For this review, take the finished solid that the model builds, in its own axes (mm). A direction names the side the tool comes from. Round coordinates to 2 decimals unless told otherwise and drop trailing zeros. Order: outer loops, then holes, each group sorted by start corner. A loop starts at its lowest first (then second) coordinate and runs counter-clockwise, first axis right, second up. Notation, with made-up numbers: (80.5, -10) -> (132.5, -10) arc R24 cw to (132.5, 3) -> close; hole circle Ø6 at (-32.75, 81.5). An arc over 180 degrees is marked (long way). Use a Markdown table: item, result. Add a question column.
1) Draft analysis for pull direction Y (two halves, no side actions). For faces 5 (the face through (29.65, 0, 16)), 6 (the face through (0, -18.5, 16)), 7 (the face through (-32, 0, 16)), state which applies: pulls with the +Y half, pulls with the -Y half, needs draft (parallel to the pull), parting line crosses it, or undercut.
2) Consider section B-B (z = 37). State the section outline as (x, y) points, plus the area to 3 significant figures.
3) Machinability: for faces 1 (the face through (30.841, 0.199, 15.496)), 2 (the face through (0, 0, 27)), 3 (the face through (-14, 17, 39)), 4 (the face through (31, 2, 2)), which of the approach directions +Z, -Z, +X, -X, +Y, -Y give a long, thin tool a straight path to every point of the face, cutting with its end or side? Answer none if there is none.
4) Wall thickness on line 1 along X through (y, z) = (12.5, 30.25); line 2 along X through (y, z) = (-12, 30); line 3 along Y through (x, z) = (-3, 19): over which ranges is each line inside the solid? List them lowest first. Write a range as [from, to].
5) Clearance check with flat-ended pins moving along their axes: P1, Ø1.5, axis at x = -11.5, y = -12, coming from the -Z side; P2, Ø2.5, axis at x = 30.5, y = 0, coming from the +Z side; P3, Ø3, axis at x = 14, y = 16, coming from the +Z side. State where each tip first meets the part, or that it passes through.
6) Consider section D-D (y = -8). State the section outline as (x, z) points.
7) Consider section C-C (z = 10). State the section outline as (x, y) points.
8) Consider section A-A (x = 17). State the section outline as (y, z) points.
```python
from build123d import *

# Parameters (mm, degrees)
SKETCH_1_W                 = 64
SKETCH_1_H                 = 37
EXTRUDE_1_DEPTH            = 42
SHELL_1_T                  = -2.35
SHELL_1_THICKNESS_2_FACE_W = 59.3
SHELL_1_THICKNESS_2_FACE_H = 32.3
SHELL_1_THICKNESS_2_DEPTH  = 12.65
F_3_0MM_START              = 27
F_3_0MM_1_OUTLINE_R        = 1.3
F_3_0MM_1_DEPTH            = 15
SKETCH_4_R                 = 18
CUT_EXTRUDE_1_DEPTH        = 79.754364958
SKETCH_5_W                 = 22
SKETCH_5_H                 = 5
CUT_EXTRUDE_2_DEPTH        = 65.474801394
SKETCH_6_R                 = 5.5
SKETCH_6_W                 = 5
SKETCH_6_H                 = 12
CUT_EXTRUDE_3_DEPTH        = 10
CUT_EXTRUDE_1_2_DEPTH      = 79.754365093
CUT_EXTRUDE_1_2_DEPTH_BACK = 10
SKETCH_7_W                 = 5
SKETCH_7_H                 = 4
FILLET_1_R                 = 2
FILLET_2_R                 = 2
FILLET_3_R                 = 0.5


# Read off the part's stored shape, not the designer's step: Ø3.0mm 暗销孔1
with BuildPart() as part:
    # 草图1 → 凸台-拉伸1 (new body)
    with BuildSketch(Plane.XY):
        Rectangle(SKETCH_1_W, SKETCH_1_H)
    extrude(amount=EXTRUDE_1_DEPTH)

    # 抽壳1
    shell_1_openings = [part.faces().sort_by_distance(p)[0] for p in [
        (0, 0, 0),
    ]]
    offset(amount=SHELL_1_T, openings=shell_1_openings, kind=Kind.INTERSECTION)

    # 抽壳1 thickness 2 face (on inner face of the shell) → 抽壳1 thickness 2 (add)
    with BuildSketch(Plane.XY.offset(39.65)):
        Rectangle(SHELL_1_THICKNESS_2_FACE_W, SHELL_1_THICKNESS_2_FACE_H)
    extrude(amount=-SHELL_1_THICKNESS_2_DEPTH)

    # Ø3.0mm 暗销孔1 outline → Ø3.0mm 暗销孔1 (cut)
    with BuildSketch(Plane.XY.offset(F_3_0MM_START)):
        with Locations((26.25, -12.5)):
            Circle(F_3_0MM_1_OUTLINE_R)
        with Locations((-26.25, 12.5)):
            Circle(F_3_0MM_1_OUTLINE_R)
        with Locations((-26.25, -12.5)):
            Circle(F_3_0MM_1_OUTLINE_R)
        with Locations((26.25, 12.5)):
            Circle(F_3_0MM_1_OUTLINE_R)
    extrude(amount=F_3_0MM_1_DEPTH, mode=Mode.SUBTRACT)

    # 草图4 → Cut-Extrude 1 (cut, through all)
    with BuildSketch(Plane(origin=(32, 0, 0), x_dir=(0, 0, -1), z_dir=(1, 0, 0))):
        with Locations((-47, 0)):
            Circle(SKETCH_4_R)
    extrude(amount=-CUT_EXTRUDE_1_DEPTH, mode=Mode.SUBTRACT)

    # 草图5 → 切除-拉伸2 (cut, through all)
    with BuildSketch(Plane.XZ.offset(18.5)):
        with Locations((14, 36.5)):
            Rectangle(SKETCH_5_W, SKETCH_5_H)
        with Locations((-14, 36.5)):
            Rectangle(SKETCH_5_W, SKETCH_5_H)
    extrude(amount=-CUT_EXTRUDE_2_DEPTH, mode=Mode.SUBTRACT)

    # 草图6 → 切除-拉伸3 (cut)
    with BuildSketch(Plane(origin=(32, 0, 0), x_dir=(0, 0, -1), z_dir=(1, 0, 0))):
        with Locations(Location((-10, 0, 0), (0, 0, 90))):
            Circle(SKETCH_6_R)
        with Locations((-22.5, 0)):
            Rectangle(SKETCH_6_W, SKETCH_6_H)
    extrude(amount=-CUT_EXTRUDE_3_DEPTH, mode=Mode.SUBTRACT)

    # 草图7 → Cut-Extrude 1 2 (cut, two sides: drawn at the far end of the back side and taken through both)
    with BuildSketch(Plane(origin=(32, 0, 0), x_dir=(0, 0, -1), z_dir=(1, 0, 0)).offset(-CUT_EXTRUDE_1_2_DEPTH_BACK)):
        with Locations((-2.5, 0)):
            Rectangle(SKETCH_7_W, SKETCH_7_H)
    extrude(amount=CUT_EXTRUDE_1_2_DEPTH + CUT_EXTRUDE_1_2_DEPTH_BACK, mode=Mode.SUBTRACT)

    # 圆角1
    fillet_1_edges = [part.edges().sort_by_distance(p)[0] for p in [
        (30.825, -6, 25),
        (30.825, 6, 25),
        (30.825, 6, 20),
        (30.825, -6, 20),
        (30.825, -2, 4.876524617),
        (30.825, 2, 4.876524617),
    ]]
    fillet(fillet_1_edges, radius=FILLET_1_R)

    # 圆角2
    # the kernel refuses this fillet: 2 mm, written as the material it takes off along each edge
    with BuildSketch(Plane(origin=(-35.388469359, -17.291616466, 42), x_dir=(0, -1.0, -4.0690356929386436e-12), z_dir=(1, 0, 0))) as fillet_2_piece_1:
        with BuildLine():
            CenterArc((1.448789292, 1.985498696), FILLET_2_R, 200.442973307, 62.653215254)
            Line((-0.425251284, 1.286948826), (-0.462732095, 1.272977829))
            ThreePointArc((-0.462732095, 1.272977829), (-0.238488291, 0.634928522), (-0.038425814, -0.011111111))
            Line((-0.038425814, -0.011111111), (0, -0.04))
            ThreePointArc((0, -0.04), (0.604191767, -0.04), (1.203575419, -0.039709974))
            Line((1.203575419, -0.039709974), (1.208383534, 0))
        make_face()
    extrude(amount=70.776938719, mode=Mode.SUBTRACT)
    with BuildSketch(Plane(origin=(-35.388469359, 17.291616466, 42), x_dir=(0, -0.31374880411831046, -0.9495060231058727), z_dir=(1, 0, 0))) as fillet_2_piece_2:
        with BuildLine():
            CenterArc((1.430687063, 1.998582), FILLET_2_R, 205.189108199, 62.653215254)
            Line((-0.379128889, 1.147367444), (-0.415325208, 1.130343153))
            ThreePointArc((-0.415325208, 1.130343153), (-0.227544685, 0.56113377), (-0.037980241, -0.012549952))
            Line((-0.037980241, -0.012549952), (0.001505986, -0.03997164))
            ThreePointArc((0.001505986, -0.03997164), (0.677693872, -0.027238004), (1.353881757, -0.03997164))
            Line((1.353881757, -0.03997164), (1.355387744, 0))
        make_face()
    extrude(amount=70.776938719, mode=Mode.SUBTRACT)

    # 圆角3
    fillet_3_edges = [part.edges().sort_by_distance(p)[0] for p in [
        (0, -18.5, 42),
        (0, 18.5, 42),
    ]]
    fillet(fillet_3_edges, radius=FILLET_3_R)


solid = part.part
```
Results list:
| question | item | result |
|---|---|---|
| 1 | face 5 | undercut |
| 1 | face 6 | pulls with the -Y half |
| 1 | face 7 | needs draft |
| 2 | outline | (-32, -18.5) -> (-25, -18.5) -> (-25, -14.97) -> (-32, -14.97) -> close; (-32, 14.97) -> (-25, 14.97) -> (-25, 18.5) -> (-32, 18.5) -> close; (-3, -18.5) -> (3, -18.5) -> (3, -14.97) -> (-3, -14.97) -> close; (-3, 14.97) -> (3, 14.97) -> (3, 18.5) -> (-3, 18.5) -> close; (25, -18.5) -> (32, -18.5) -> (32, -14.97) -> (25, -14.97) -> close; (25, 14.97) -> (32, 14.97) -> (32, 18.5) -> (25, 18.5) -> close |
| 2 | area | 141 mm2 |
| 3 | face 1 | +X |
| 3 | face 2 | -Z |
| 3 | face 3 | +Y, -Y |
| 3 | face 4 | -Z, +X |
| 4 | line 1 | [-32, -27.55], [-24.95, 24.95], [27.55, 32] |
| 4 | line 2 | [-32, -27.45], [-25.05, 25.05], [27.45, 32] |
| 4 | line 3 | [-18.5, -16.15], [16.15, 18.5] |
| 5 | P1 | z = 27 |
| 5 | P2 | z = 29.04 |
| 5 | P3 | z = 41.58 |
| 6 | outline | (-32, 0) -> (-29.65, 0) -> (-29.65, 27) -> (29.65, 27) -> (29.65, 0) -> (32, 0) -> (32, 30.88) -> (-32, 30.88) -> close |
| 7 | outline | (-32, -18.5) -> (32, -18.5) -> (32, -5.5) -> (29.65, -5.5) -> (29.65, -16.15) -> (-29.65, -16.15) -> (-29.65, 16.15) -> (29.65, 16.15) -> (29.65, 5.5) -> (32, 5.5) -> (32, 18.5) -> (-32, 18.5) -> close |
| 8 | outline | (-18.5, 0) -> (-16.15, 0) -> (-16.15, 27) -> (16.15, 27) -> (16.15, 0) -> (18.5, 0) -> (18.5, 34) -> (12.45, 34) arc R18 cw to (-12.45, 34) -> (-18.5, 34) -> close; (-18.5, 39) -> (-16.12, 39) arc R18 cw to (-16.87, 40.71) arc R2 ccw to (-17.75, 41.75) arc R0.5 ccw to (-18.5, 41.32) -> close; (16.12, 39) -> (18.5, 39) -> (18.5, 41.32) arc R0.5 ccw to (17.75, 41.75) arc R2 ccw to (16.87, 40.71) arc R18 cw to start |
